```python
from build123d import *

# Parameters (mm, degrees)
BOSS_EXTRUDE1_DEPTH             = 49
CHAMFER1_SIZE                   = 1
M8_TAPPED_HOLE1_D               = 6.8
M8_TAPPED_HOLE1_DEPTH           = 19.75
M8_TAPPED_HOLE1_TIP             = 2.042926105
M8_TAPPED_HOLE1_ON_FACE_2_D     = 6.8
M8_TAPPED_HOLE1_ON_FACE_2_DEPTH = 19.75
M8_TAPPED_HOLE1_ON_FACE_2_TIP   = 2.042926105
CUT_EXTRUDE1_START              = 10
CUT_EXTRUDE1_DEPTH              = 3.5


with BuildPart() as part:
    # Sketch1 → Boss-Extrude1 (new, symmetric)
    with BuildSketch(Plane.XY):
        with BuildLine():
            ThreePointArc((0.789917583, 13.977697601), (0, 14), (-0.789917583, 13.977697601))
            Line((-0.789917583, 13.977697601), (-11.710082417, 7.672937494))
            ThreePointArc((-11.710082417, 7.672937494), (-12.124355653, 7), (-12.5, 6.304760106))
            Line((-12.5, 6.304760106), (-12.5, -6.304760106))
            ThreePointArc((-12.5, -6.304760106), (-12.124355653, -7), (-11.710082417, -7.672937494))
            Line((-11.710082417, -7.672937494), (-0.789917583, -13.977697601))
            ThreePointArc((-0.789917583, -13.977697601), (0, -14), (0.789917583, -13.977697601))
            Line((0.789917583, -13.977697601), (11.710082417, -7.672937494))
            ThreePointArc((11.710082417, -7.672937494), (12.124355653, -7), (12.5, -6.304760106))
            Line((12.5, -6.304760106), (12.5, 6.304760106))
            ThreePointArc((12.5, 6.304760106), (12.124355653, 7), (11.710082417, 7.672937494))
            Line((11.710082417, 7.672937494), (0.789917583, 13.977697601))
        make_face()
    extrude(amount=BOSS_EXTRUDE1_DEPTH, both=True)

    # Sketch2 → Revolve1 (revolve)
    with BuildSketch(Plane(origin=(0, 0, 0), x_dir=(0, 0, -1), z_dir=(1, 0, 0)), mode=Mode.PRIVATE) as revolve1_sk:
        Polygon((-93, 0), (-93, 10), (-52, 10), (-52, 12.5), (-49, 12.5), (-49, 0), align=None)
        Polygon((52, 10), (64, 10), (64, 0), (49, 0), (49, 12.5), (52, 12.5), align=None)
    revolve(revolve1_sk.sketch.rotate(Axis((0, 0, -70.752525622), (0, 0, 1)), 90), axis=Axis((0, 0, -70.752525622), (0, 0, 1)))

    # Chamfer1
    chamfer1_edges = [part.edges().sort_by_distance(p)[0] for p in [
        (10, 0, 93),
        (10, 0, -64),
    ]]
    chamfer(chamfer1_edges, length=CHAMFER1_SIZE)

    # M8 Tapped Hole1
    with Locations(Plane.XY.offset(93)):
        with Locations((0, 0)):
            Hole(M8_TAPPED_HOLE1_D / 2, depth=M8_TAPPED_HOLE1_DEPTH)
            with Locations((0, 0, -(M8_TAPPED_HOLE1_DEPTH + M8_TAPPED_HOLE1_TIP / 2))):  # 118° drill point
                Cone(0, M8_TAPPED_HOLE1_D / 2, M8_TAPPED_HOLE1_TIP, mode=Mode.SUBTRACT)

    # M8 Tapped Hole1 on face 2
    with Locations(Plane(origin=(0, 0, -64), x_dir=(-1, 0, 0), z_dir=(0, 0, -1))):
        with Locations((0, 0)):
            Hole(M8_TAPPED_HOLE1_ON_FACE_2_D / 2, depth=M8_TAPPED_HOLE1_ON_FACE_2_DEPTH)
            with Locations((0, 0, -(M8_TAPPED_HOLE1_ON_FACE_2_DEPTH + M8_TAPPED_HOLE1_ON_FACE_2_TIP / 2))):  # 118° drill point
                Cone(0, M8_TAPPED_HOLE1_ON_FACE_2_D / 2, M8_TAPPED_HOLE1_ON_FACE_2_TIP, mode=Mode.SUBTRACT)

    # Sketch4 → Cut-Extrude1 (cut)
    with BuildSketch(Plane(origin=(0, 0, 0), x_dir=(0, 0, -1), z_dir=(1, 0, 0)).offset(CUT_EXTRUDE1_START)):
        with BuildLine():
            Line((-93, -3), (-71, -3))
            ThreePointArc((-71, -3), (-68, 0), (-71, 3))
            Line((-71, 3), (-93, 3))
            ThreePointArc((-93, 3), (-96, 0), (-93, -3))
        make_face()
    extrude(amount=-CUT_EXTRUDE1_DEPTH, mode=Mode.SUBTRACT)


solid = part.part
```
Design review of the part built by this model. Coordinates are the model's own, in mm. A direction names the side the tool comes from. Coordinates: 2 decimals unless noted, no trailing zeros. Loops run counter-clockwise (first coordinate to the right, second up) from the corner with the lowest first, then second, coordinate; pieces in that order, holes last. Notation, with made-up numbers: (35.25, 30) -> (73.25, 30) arc R33 ccw to (73.25, 59) -> close; hole circle Ø6 at (59.25, 59). An arc over 180 degrees is marked (long way). Answer as a JSON object with one key per item and string values.
Q1. Take a section at A-A on z = 47. Give the boundary of the cut face in (x, y), plus the area to 3 significant figures.
Answer block:
{"outline": "(-12.5, -6.3) arc R14 ccw to (-11.71, -7.67) -> (-0.79, -13.98) arc R14 ccw to (0.79, -13.98) -> (11.71, -7.67) arc R14 ccw to (12.5, -6.3) -> (12.5, 6.3) arc R14 ccw to (11.71, 7.67) -> (0.79, 13.98) arc R14 ccw to (-0.79, 13.98) -> (-11.71, 7.67) arc R14 ccw to (-12.5, 6.3) -> close", "area": "539 mm^2"}
Q2. Tool access review of faces 1 (the flat face through (-11.2, 6.2, 49)), 2 (the flat face through (0.1, -10.2, -52)), 3 (the flat face through (11.2, 6.2, 49)), 4 (the flat face through (11, -7, -49)), 5 (the flat face through (-11, -7, 49)): name each direction out of +Z, -Z, +X, -X, +Y, -Y from which nothing blocks a thin tool from reaching the whole face with its end or side.
Answer block:
{"face 1": "+Z, -X, +Y", "face 2": "-Z", "face 3": "+Z, +X, +Y", "face 4": "-Z, +X, -Y", "face 5": "+Z, -X, -Y"}
Q3. The part is to be moulded in two halves that separate along Y. For faces 6 (the flat face through (0, -13, 49)), 7 (the flat face through (6.5, 0, 81)), 8 (the cylindrical face through (-11.923, -3.755, -50.521)), say which applies: +Y half, -Y half, draft (parallel to the pull), parting line (faces both ways), or undercut.
Answer block:
{"face 6": "draft", "face 7": "undercut", "face 8": "parting line"}
Q4. Clearance check with flat-ended pins moving along their axes: pin 1 Ø1 at (x, y) = (-1, -0.5) entering from +Z; pin 2 Ø2.5 at (x, y) = (2.5, -11.5) entering from +Z; pin 3 Ø3 at (x, z) = (-7.5, 36) entering from -Y. State where each tip first meets the part, or that it passes through.
Answer block:
{"pin 1": "stops at z = 72.18", "pin 2": "stops at z = 52", "pin 3": "stops at y = -10.97"}
Q5. To check wall thickness, follow L1, parallel to Y at x = 0, z = 88; L2, parallel to Z at x = -2.75, y = -11.75; L3, parallel to Z at x = 2.5, y = -1.75. State the ranges of each line that lie inside material, in increasing order.
Answer block:
{"L1": "y = -10 to -3.4, 3.4 to 10", "L2": "z = -52 to 52", "L3": "z = -44.04 to 73.04"}
